Geometry check sheet. Reference: the model listing, model coordinates, mm. A direction names the side the tool comes from. Give positions to 0.01 mm unless a question says otherwise; leave off trailing zeros. Loops run counter-clockwise (first coordinate to the right, second up) from the corner with the lowest first, then second, coordinate; pieces in that order, holes last.
1. Cross-section at B-B, the plane x = 15.5. Record the cut outline in (y, z).
2. Release check for a two-part mould opening along Y. For faces 4 (the flat face through (30.535, 10.607, 54.505)), 5 (the cylindrical face through (-7.96, -12.65, -8.06)), 6 (the flat face through (30.535, 52.506, 18.067)) record: +Y half, -Y half, draft (parallel to the pull), parting line (faces both ways), or undercut.
3. Material ranges on L1, parallel to Y at x = -2, z = -26; L2, parallel to X at y = 1, z = 2.5; L3, parallel to Y at x = 0.5, z = -7.5, recorded low to high.
4. Tool access check on faces 1 (the cylindrical face through (30.465, -49.284, -8.629)), 2 (the flat face through (30.535, -52.317, 18.296)), 3 (the flat face through (-2.465, 19.845, -34.442)). Record the directions out of +Z, -Z, +X, -X, +Y, -Y that give a thin tool (end or side, any length) a straight path to the whole face; none if there is none.
5. Go/stop test with flat-tipped pins: pin 1 Ø12 at (x, z) = (17.5, -43.5) entering from +Y; pin 2 Ø12 at (x, z) = (3.5, 3.5) entering from +Y; pin 3 Ø7.5 at (y, z) = (28, 0) entering from -X. Record where each tip stops, or that it passes through.
6. Cross-section at A-A, the plane x = -6.5. Record the cut outline in (y, z).
from build123d import *

# Parameters (mm, degrees)
SKETCH2_R           = 2.05
CUT_EXTRUDE1_DEPTH  = 10
SKETCH5_R           = 24.5
CUT_EXTRUDE4_DEPTH  = 2
BOSS_EXTRUDE1_DEPTH = 5
CIRPATTERN2_COUNT   = 6
CHAMFER2_SIZE       = 5.5
CHAMFER3_SIZE       = 1.5
SKETCH9_R           = 15
BOSS_EXTRUDE2_DEPTH = 7
CHAMFER4_SIZE       = 1
CUT_EXTRUDE7_START  = -5
CUT_EXTRUDE7_DEPTH  = 5
SKETCH12_R          = 3.25
CUT_EXTRUDE8_DEPTH  = 5


with BuildPart() as part:
    # Sketch1 → Revolve1 (revolve)
    with BuildSketch(Plane.XY, mode=Mode.PRIVATE) as revolve1_sk:
        Polygon((-5, 0), (-5, 52), (33, 52), (33, 47), (0, 47), (0, 0), align=None)
    revolve(revolve1_sk.sketch.rotate(Axis((-58.663171691, 0, 0), (1, 0, 0)), 90), axis=Axis((-58.663171691, 0, 0), (1, 0, 0)))

    # Sketch2 → Cut-Extrude1 (cut)
    with BuildSketch(Plane(origin=(0, 0, 0), x_dir=(0, 0, -1), z_dir=(1, 0, 0))):
        with Locations((0, 28)):
            Circle(SKETCH2_R)
        with Locations((24.248711306, 14)):
            Circle(SKETCH2_R)
        with Locations((24.248711306, -14)):
            Circle(SKETCH2_R)
        with Locations((0, -28)):
            Circle(SKETCH2_R)
        with Locations((-24.248711306, -14)):
            Circle(SKETCH2_R)
        with Locations((-24.248711306, 14)):
            Circle(SKETCH2_R)
        with BuildLine():
            Line((-2.5, 44.75), (2.5, 44.75))
            ThreePointArc((2.5, 44.75), (5, 42.25), (2.5, 39.75))
            Line((2.5, 39.75), (-2.5, 39.75))
            ThreePointArc((-2.5, 39.75), (-5, 42.25), (-2.5, 44.75))
        make_face()
    cut_extrude1 = extrude(amount=-CUT_EXTRUDE1_DEPTH, mode=Mode.SUBTRACT)

    # Sketch5 → Cut-Extrude4 (cut)
    with BuildSketch(Plane(origin=(0, 0, 0), x_dir=(0, 0, -1), z_dir=(1, 0, 0))):
        Circle(SKETCH5_R)
    extrude(amount=-CUT_EXTRUDE4_DEPTH, mode=Mode.SUBTRACT)

    # Sketch6 → Boss-Extrude1 (add)
    with BuildSketch(Plane(origin=(33, 0, 0), x_dir=(0, 0, -1), z_dir=(1, 0, 0))):
        Polygon((-10, 59.160797831), (-26.363112951, 45.662251077), (-46.23475383, 38.240652953), (-56.23475383, 20.920144878), (-52.726225902, 0), (-56.23475383, -20.920144878), (-46.23475383, -38.240652953), (-26.363112951, -45.662251077), (-10, -59.160797831), (10, -59.160797831), (26.363112951, -45.662251077), (46.23475383, -38.240652953), (56.23475383, -20.920144878), (52.726225902, 0), (56.23475383, 20.920144878), (46.23475383, 38.240652953), (26.363112951, 45.662251077), (10, 59.160797831), align=None)
        with BuildLine():
            ThreePointArc((-51.283776788, 8.600827774), (-45.033320997, 26), (-33.09042374, 40.112639613))
            ThreePointArc((-33.09042374, 40.112639613), (-26, 45.033320997), (-18.193353048, 48.713467387))
            ThreePointArc((-18.193353048, 48.713467387), (0, 52), (18.193353048, 48.713467387))
            ThreePointArc((18.193353048, 48.713467387), (26, 45.033320997), (33.09042374, 40.112639613))
            ThreePointArc((33.09042374, 40.112639613), (45.033320997, 26), (51.283776788, 8.600827774))
            ThreePointArc((51.283776788, 8.600827774), (51.820634852, 4.315298776), (52, 0))
            ThreePointArc((52, 0), (51.820634852, -4.315298776), (51.283776788, -8.600827774))
            ThreePointArc((51.283776788, -8.600827774), (45.033320997, -26), (33.09042374, -40.112639613))
            ThreePointArc((33.09042374, -40.112639613), (26, -45.033320997), (18.193353048, -48.713467387))
            ThreePointArc((18.193353048, -48.713467387), (0, -52), (-18.193353048, -48.713467387))
            ThreePointArc((-18.193353048, -48.713467387), (-26, -45.033320997), (-33.09042374, -40.112639613))
            ThreePointArc((-33.09042374, -40.112639613), (-45.033320997, -26), (-51.283776788, -8.600827774))
            ThreePointArc((-51.283776788, -8.600827774), (-52, 0), (-51.283776788, 8.600827774))
        make_face(mode=Mode.SUBTRACT)
    extrude(amount=-BOSS_EXTRUDE1_DEPTH)

    # CirPattern2: Cut-Extrude1 ×6 about axis
    cirpattern2_axis = Axis((0, 0, 0), (1, 0, 0))
    for i in range(1, CIRPATTERN2_COUNT):
        add(cut_extrude1.rotate(cirpattern2_axis, i * 360 / CIRPATTERN2_COUNT), mode=Mode.SUBTRACT)

    # Chamfer2
    chamfer2_edges = [part.edges().sort_by_distance(p)[0] for p in [
        (-5, 0, -52),
    ]]
    chamfer(chamfer2_edges, length=CHAMFER2_SIZE)

    # Chamfer3
    # the kernel refuses this chamfer: 1.5 mm, written as the material it takes off along each edge
    with BuildSketch(Plane(origin=(0, 0, 0), x_dir=(0, 0, -1), z_dir=(0, -1, 0))) as chamfer3_piece_1:
        Polygon((24.5 + CHAMFER3_SIZE, 0), (24.5, -CHAMFER3_SIZE), (24.5, 0), align=None)
    revolve(axis=Axis((0, 0, 0), (1, 0, 0)), mode=Mode.SUBTRACT)

    # Sketch9 → Boss-Extrude2 (add)
    with BuildSketch(Plane.ZY.offset(5)):
        with Locations(Location((0, 0, 0), (0, 0, 180))):
            Circle(SKETCH9_R)
    extrude(amount=BOSS_EXTRUDE2_DEPTH)

    # Chamfer4
    chamfer4_edges = [part.edges().sort_by_distance(p)[0] for p in [
        (-12, 0, 15),
    ]]
    chamfer(chamfer4_edges, length=CHAMFER4_SIZE)

    # Sketch11 → Cut-Extrude7 (cut)
    with BuildSketch(Plane(origin=(33, 0, 0), x_dir=(0, 0, -1), z_dir=(1, 0, 0)).offset(CUT_EXTRUDE7_START)):
        with BuildLine():
            ThreePointArc((-9.948403245, 45.935054946), (-8.16146435, 46.285964392), (-6.362272958, 46.567386472))
            ThreePointArc((-6.362272958, 46.567386472), (-8.68848657, 49.274855922), (-9.948403245, 45.935054946))
        make_face()
        with BuildLine():
            ThreePointArc((9.948403245, 45.935054946), (8.68848657, 49.274855922), (6.362272958, 46.567386472))
            ThreePointArc((6.362272958, 46.567386472), (8.16146435, 46.285964392), (9.948403245, 45.935054946))
        make_face()
        with BuildLine():
            ThreePointArc((25.059155194, 39.762277864), (25.0175, 43.331581078), (21.905565146, 41.583003928))
            ThreePointArc((21.905565146, 41.583003928), (23.5, 40.703193978), (25.059155194, 39.762277864))
        make_face()
        with BuildLine():
            ThreePointArc((37.147403193, 28.793583244), (38.329033711, 32.161878051), (34.806722885, 31.58309741))
            ThreePointArc((34.806722885, 31.58309741), (36.004088827, 30.211017655), (37.147403193, 28.793583244))
        make_face()
        with BuildLine():
            ThreePointArc((44.75512613, 14.351957536), (47.017520281, 17.112977871), (43.509676151, 17.773803228))
            ThreePointArc((43.509676151, 17.773803228), (44.165553177, 16.074946736), (44.75512613, 14.351957536))
        make_face()
        with BuildLine():
            ThreePointArc((46.96472034, -1.820726063), (50.035, 0), (46.96472034, 1.820726063))
            ThreePointArc((46.96472034, 1.820726063), (46.991179257, 0.910533917), (47, 0))
            ThreePointArc((47, 0), (46.991179257, -0.910533917), (46.96472034, -1.820726063))
        make_face()
        with BuildLine():
            ThreePointArc((43.509676151, -17.773803228), (47.017520281, -17.112977871), (44.75512613, -14.351957536))
            ThreePointArc((44.75512613, -14.351957536), (44.165553177, -16.074946736), (43.509676151, -17.773803228))
        make_face()
        with BuildLine():
            ThreePointArc((34.806722885, -31.58309741), (38.329033711, -32.161878051), (37.147403193, -28.793583244))
            ThreePointArc((37.147403193, -28.793583244), (36.004088827, -30.211017655), (34.806722885, -31.58309741))
        make_face()
        with BuildLine():
            ThreePointArc((21.905565146, -41.583003928), (25.0175, -43.331581078), (25.059155194, -39.762277864))
            ThreePointArc((25.059155194, -39.762277864), (23.5, -40.703193978), (21.905565146, -41.583003928))
        make_face()
        with BuildLine():
            ThreePointArc((6.362272958, -46.567386472), (8.68848657, -49.274855922), (9.948403245, -45.935054946))
            ThreePointArc((9.948403245, -45.935054946), (8.16146435, -46.285964392), (6.362272958, -46.567386472))
        make_face()
        with BuildLine():
            ThreePointArc((-6.362272958, -46.567386472), (-8.16146435, -46.285964392), (-9.948403245, -45.935054946))
            ThreePointArc((-9.948403245, -45.935054946), (-8.68848657, -49.274855922), (-6.362272958, -46.567386472))
        make_face()
        with BuildLine():
            ThreePointArc((-21.905565146, -41.583003928), (-23.5, -40.703193978), (-25.059155194, -39.762277864))
            ThreePointArc((-25.059155194, -39.762277864), (-25.0175, -43.331581078), (-21.905565146, -41.583003928))
        make_face()
        with BuildLine():
            ThreePointArc((-34.806722885, -31.58309741), (-36.004088827, -30.211017655), (-37.147403193, -28.793583244))
            ThreePointArc((-37.147403193, -28.793583244), (-38.329033711, -32.161878051), (-34.806722885, -31.58309741))
        make_face()
        with BuildLine():
            ThreePointArc((-43.509676151, -17.773803228), (-44.165553177, -16.074946736), (-44.75512613, -14.351957536))
            ThreePointArc((-44.75512613, -14.351957536), (-47.017520281, -17.112977871), (-43.509676151, -17.773803228))
        make_face()
        with BuildLine():
            ThreePointArc((-46.96472034, -1.820726063), (-47, 0), (-46.96472034, 1.820726063))
            ThreePointArc((-46.96472034, 1.820726063), (-50.035, 0), (-46.96472034, -1.820726063))
        make_face()
        with BuildLine():
            ThreePointArc((-44.75512613, 14.351957536), (-44.165553177, 16.074946736), (-43.509676151, 17.773803228))
            ThreePointArc((-43.509676151, 17.773803228), (-47.017520281, 17.112977871), (-44.75512613, 14.351957536))
        make_face()
        with BuildLine():
            ThreePointArc((-37.147403193, 28.793583244), (-36.004088827, 30.211017655), (-34.806722885, 31.58309741))
            ThreePointArc((-34.806722885, 31.58309741), (-38.329033711, 32.161878051), (-37.147403193, 28.793583244))
        make_face()
        with BuildLine():
            ThreePointArc((-25.059155194, 39.762277864), (-23.5, 40.703193978), (-21.905565146, 41.583003928))
            ThreePointArc((-21.905565146, 41.583003928), (-25.0175, 43.331581078), (-25.059155194, 39.762277864))
        make_face()
    extrude(amount=CUT_EXTRUDE7_DEPTH, mode=Mode.SUBTRACT)

    # Sketch12 → Cut-Extrude8 (cut)
    with BuildSketch(Plane.ZY.offset(5)):
        with Locations((0, 28)):
            Circle(SKETCH12_R)
        with Locations((24.248711306, 14)):
            Circle(SKETCH12_R)
        with Locations((24.248711306, -14)):
            Circle(SKETCH12_R)
        with Locations((0, -28)):
            Circle(SKETCH12_R)
        with Locations((-24.248711306, -14)):
            Circle(SKETCH12_R)
        with Locations((-24.248711306, 14)):
            Circle(SKETCH12_R)
    extrude(amount=-CUT_EXTRUDE8_DEPTH, mode=Mode.SUBTRACT)


solid = part.part
Result:
1. outline: circle Ø104 at (0, 0); hole circle Ø94 at (0, 0)
2. face 4: undercut
2. face 5: parting line
2. face 6: +Y half
3. L1: y = -42.12 to -16.74, -11.26 to 11.26, 16.74 to 42.12
3. L2: x = -12 to -2
3. L3: y = -51.46 to -46.4, 46.4 to 51.46
4. face 1: +X
4. face 2: +Z, +X, -X, -Y
4. face 3: +X, -X
5. pin 1: stops at y = 36.02
5. pin 2: stops at y = 52
5. pin 3: stops at x = -5
6. outline: circle Ø30 at (0, 0)
